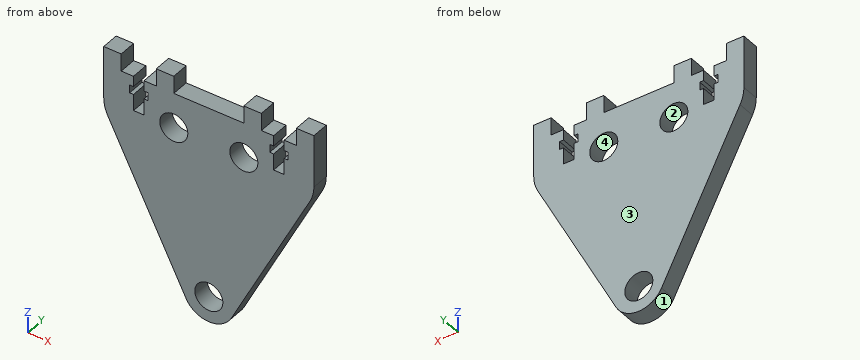
```python
from build123d import *

# Parameters (mm, degrees)
SKETCH1_R           = 4
BOSS_EXTRUDE1_DEPTH = 5


with BuildPart() as part:
    # Sketch1 → Boss-Extrude1 (new body)
    with BuildSketch(Plane(origin=(0, 0, 0), x_dir=(1, 0, 0), z_dir=(0, 1, 0))):
        with BuildLine():
            Line((-30, 10), (-30, -5))
            Line((-30, -5), (-25, -5))
            Line((-25, -5), (-25, 0))
            Line((-25, 0), (-21.5, 0))
            Line((-21.5, 0), (-21.5, 3))
            Line((-21.5, 3), (-22.6, 3))
            Line((-22.6, 3), (-22.6, 5.3))
            Line((-22.6, 5.3), (-21.5, 5.3))
            Line((-21.5, 5.3), (-21.5, 10))
            Line((-21.5, 10), (-18.5, 10))
            Line((-18.5, 10), (-18.5, 5.3))
            Line((-18.5, 5.3), (-17.4, 5.3))
            Line((-17.4, 5.3), (-17.4, 3))
            Line((-17.4, 3), (-18.5, 3))
            Line((-18.5, 3), (-18.5, 0))
            Line((-18.5, 0), (-15, 0))
            Line((-15, 0), (-15, -5))
            Line((-15, -5), (-10, -5))
            Line((-10, -5), (-10, 0))
            Line((-10, 0), (10, 0))
            Line((10, 0), (10, -5))
            Line((10, -5), (15, -5))
            Line((15, -5), (15, 0))
            Line((15, 0), (18.5, 0))
            Line((18.5, 0), (18.5, 3))
            Line((18.5, 3), (17.4, 3))
            Line((17.4, 3), (17.4, 5.3))
            Line((17.4, 5.3), (18.5, 5.3))
            Line((18.5, 5.3), (18.5, 10))
            Line((18.5, 10), (21.5, 10))
            Line((21.5, 10), (21.5, 5.3))
            Line((21.5, 5.3), (22.6, 5.3))
            Line((22.6, 5.3), (22.6, 3))
            Line((22.6, 3), (21.5, 3))
            Line((21.5, 3), (21.5, 0))
            Line((21.5, 0), (25, 0))
            Line((25, 0), (25, -5))
            Line((25, -5), (30, -5))
            Line((30, -5), (30, 10))
            ThreePointArc((30, 10), (29.721396184, 12.344025646), (28.901108754, 14.557440395))
            Line((28.901108754, 14.557440395), (6.492233497, 58.324076585))
            ThreePointArc((6.492233497, 58.324076585), (0, 62.293735732), (-6.492233497, 58.324076585))
            Line((-6.492233497, 58.324076585), (-28.901108754, 14.557440395))
            ThreePointArc((-28.901108754, 14.557440395), (-29.721396184, 12.344025646), (-30, 10))
        make_face()
        with Locations(Location((0, 55, 0), (0, 0, 90))):
            Circle(SKETCH1_R, mode=Mode.SUBTRACT)
        with Locations(Location((-10, 10, 0), (0, 0, 270))):
            Circle(SKETCH1_R, mode=Mode.SUBTRACT)
        with Locations(Location((10, 10, 0), (0, 0, 90))):
            Circle(SKETCH1_R, mode=Mode.SUBTRACT)
    extrude(amount=BOSS_EXTRUDE1_DEPTH)


solid = part.part
```
Geometry check sheet. Reference: the model listing, model coordinates, mm. Face numbers are marked on the shaded views. Give positions to 0.01 mm unless a question says otherwise; leave off trailing zeros. Write each loop counter-clockwise with the first axis right and the second up, starting at its lowest first coordinate (ties: lowest second). Pieces come first, ordered by that corner, then holes. Notation, with made-up numbers: (-2, 83) -> (8, 83) arc R28 cw to (8, 110) -> close; hole circle Ø1 at (44.5, 41). An arc over 180 degrees is marked (long way). Use one line per item in the form item = value.
Item 1: Mould release check, pull along X, two halves, no side actions. Record for the marked faces 1, 2, 3 and 4: released by +X, released by -X, zero draft, split by the parting line, or undercut.
Results list:
face_1 = split by the parting line
face_2 = undercut
face_3 = zero draft
face_4 = undercut
Item 2: Sectioned sample at C-C on y = 1.5. Count the separate pieces of the cut face and the enclosed holes in it, plus the area to 3 significant figures.
Results list:
separate_pieces = 1
enclosed_holes = 3
area = 2,340 mm2
Item 3: Depth check by flat-ended pin: pin 1 Ø0.9 at (x, y) = (19.5, 3) entering from +Z; pin 2 Ø1.5 at (x, z) = (20.5, -36.5) entering from +Y; pin 3 Ø3 at (x, y) = (-22.5, 2) entering from +Z; pin 4 Ø1.5 at (x, y) = (21.5, 2) entering from -Z. Enter the tip coordinate at first touch or a pass-through.
Results list:
pin_1 = -10
pin_2 = through
pin_3 = 0
pin_4 = -30.48
Item 4: Sectioned sample at A-A on x = 0. Enter the section's corners in (y, z).
Results list:
outline = (0, -62.29) -> (5, -62.29) -> (5, -59) -> (0, -59) -> close; (0, -51) -> (5, -51) -> (5, 0) -> (0, 0) -> close
Item 5: Scan lines: line 1 (X direction, y = 2.2, z = -11.5); line 2 (Z direction, x = 17.5, y = 4.4); line 3 (Z direction, x = -7.5, y = 1.4). Record each from-to range of solid material in increasing order.
Results list:
line_1 = -29.89 to -13.71, -6.29 to 6.29, 13.71 to 29.89
line_2 = -36.82 to -5.3, -3 to 0
line_3 = -56.36 to -13.12, -6.88 to 0
Item 6: Sectioned sample at D-D on z = -29. Enter the section's corners in (x, y).
Results list:
outline = (-21.51, 0) -> (21.51, 0) -> (21.51, 5) -> (-21.51, 5) -> close
Item 7: Sectioned sample at B-B on z = -55. Enter the section's corners in (x, y), plus the area to 3 significant figures.
Results list:
outline = (-8.19, 0) -> (-4, 0) -> (-4, 5) -> (-8.19, 5) -> close; (4, 0) -> (8.19, 0) -> (8.19, 5) -> (4, 5) -> close
area = 41.9 mm2
